```python
from build123d import *

# Parameters (mm, degrees)
BOSS_EXTRUDE1_DEPTH = 5
CUT_EXTRUDE1_START  = -10
CUT_EXTRUDE1_DEPTH  = 10


with BuildPart() as part:
    # Sketch1 → Boss-Extrude1 (new body)
    with BuildSketch(Plane(origin=(0, 0, 0), x_dir=(1, 0, 0), z_dir=(0, 1, 0))):
        with BuildLine():
            Line((0, 0), (8, 0))
            Line((8, 0), (8, -37))
            ThreePointArc((8, -37), (-0.020288742, -67.450779957), (-22, -90))
            ThreePointArc((-22, -90), (-5.718469366, -65.692333471), (0, -37))
            Line((0, -37), (0, -8))
            Line((0, -8), (0, 0))
        make_face()
    extrude(amount=BOSS_EXTRUDE1_DEPTH)

    # Sketch2 → Cut-Extrude1 (cut)
    with BuildSketch(Plane(origin=(0, 5, 0), x_dir=(1, 0, 0), z_dir=(0, 1, 0)).offset(CUT_EXTRUDE1_START)):
        with BuildLine():
            Line((-10.364854051, -75), (-5.059100302, -75))
            ThreePointArc((-5.059100302, -75), (-12.837382179, -83.28172988), (-22, -90))
            ThreePointArc((-22, -90), (-15.704900448, -82.870406095), (-10.364854051, -75))
        make_face()
    extrude(amount=CUT_EXTRUDE1_DEPTH, mode=Mode.SUBTRACT)


solid = part.part
```
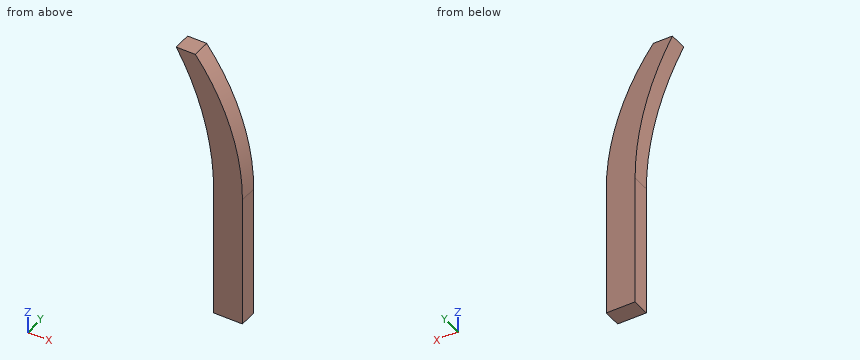
Part model, mm, in its own coordinate system. Round coordinates to 2 decimals unless told otherwise and drop trailing zeros. Write each loop counter-clockwise with the first axis right and the second up, starting at its lowest first coordinate (ties: lowest second). Pieces come first, ordered by that corner, then holes.
Item 1: Drop flat-ended pins along their axis: pin 1 Ø4 at (x, z) = (-4, 59.5) entering from +Y; pin 2 Ø2.5 at (y, z) = (2.5, 9.5) entering from -X. Give the stop position or say it passes through.
Results:
pin 1: stops at y = 5
pin 2: stops at x = 0
Item 2: Probe L1, parallel to X at y = 4.05, z = 32.5; L2, parallel to X at y = 3.7, z = 69; L3, parallel to Z at x = -6, y = 4.75. List the from-to ranges inside material, lowest first.
Results:
L1: x = 0 to 8
L2: x = -7.19 to -0.93
L3: z = 66.36 to 75
Item 3: Cut at B-B, the plane z = 35. Give the cut face in (x, y).
Results:
outline: (0, 0) - (8, 0) - (8, 5) - (0, 5) - close
Item 4: Cut at C-C, the plane x = -2.5. Give the cut face in (y, z).
Results:
outline: (0, 56.18) - (5, 56.18) - (5, 71.47) - (0, 71.47) - close
Item 5: Cut at A-A, the plane y = 2.6. Give the cut face in (x, z).
Results:
outline: (-10.36, 75) arc R74.84 cw to (0, 37) - (0, 0) - (8, 0) - (8, 37) arc R61.82 ccw to (-5.06, 75) - close
